Study the drawing (mm; zero at the part's minimum x, y, z) and answer. Give positions to 0.01 mm unless a question says otherwise; leave off trailing zeros. Write each loop counter-clockwise with the first axis right and the second up, starting at its lowest first coordinate (ties: lowest second). Pieces come first, ordered by that corner, then holes. Notation, with made-up numbers: (3, -38) -> (54, -38) arc R16 ccw to (54, -17) -> close; hole circle Ø8 at (44.25, 34.25). An arc over 180 degrees is marked (long way). Put each result on its own line as item: value. Start each with the question number.
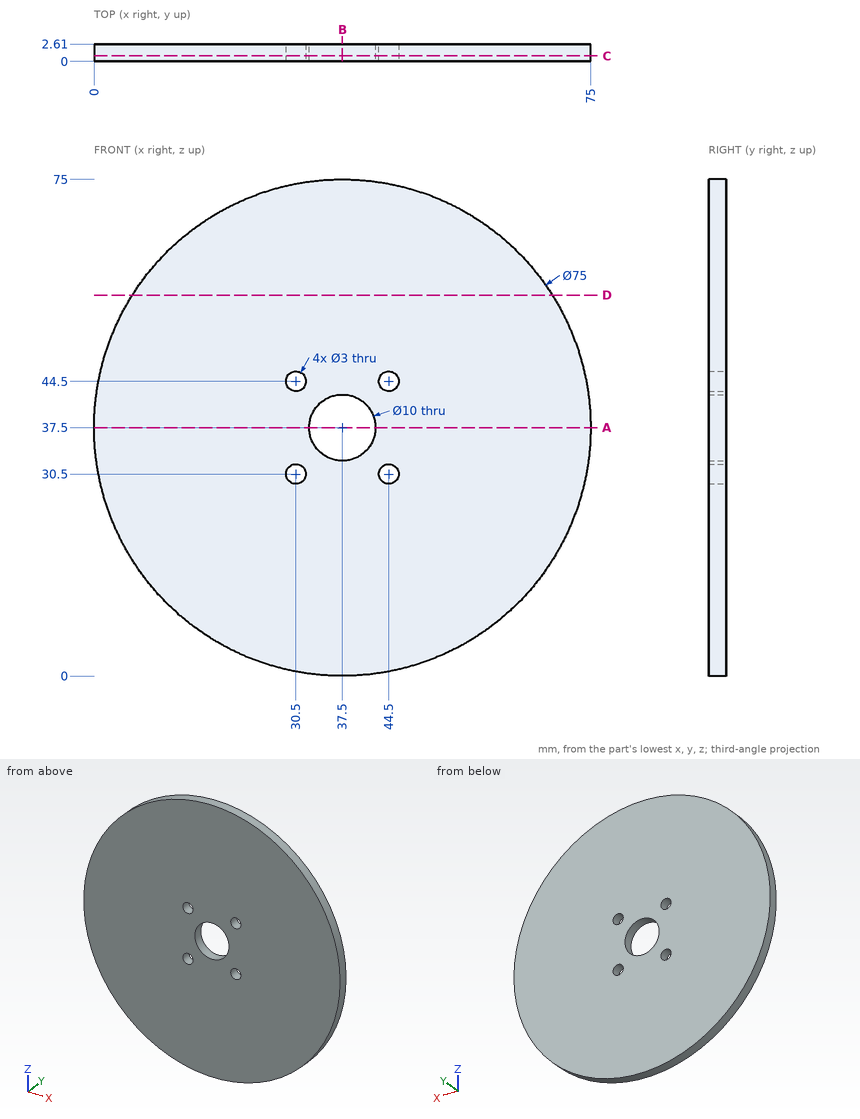
1) A cutting plane is placed at A-A on z = 37.5. Give the vertices of the cut face in (x, y), and give its area (3 significant figures).
2) A cutting plane is placed at C-C on y = 0.8. Give the vertices of the cut face in (x, z), and give its area (3 significant figures).
3) Straight lines are drawn through the part: line 1 (Z direction, x = 30.5, y = 1.15); line 2 (X direction, y = 1.1, z = 37.5). For each, find the intervals that lie inside material, in ascending order. Write a range as [from, to].
4) A cutting plane is placed at D-D on z = 57.5. Give the vertices of the cut face in (x, y), and give its area (3 significant figures).
5) A cutting plane is placed at B-B on x = 37.5. Give the vertices of the cut face in (y, z).
6) Each of these flat-tipped pins is pushed along its axis until it touches: pin 1 Ø1.5 at (y, z) = (2, 56.5) entering from -X; pin 2 Ø1.5 at (x, y) = (16.5, 1.5) entering from -Z; pin 3 Ø1.5 at (y, z) = (1.5, 35.5) entering from -X. Where does it stop, or does it pass through?
Results found:
1. outline: (0, 0) -> (32.5, 0) -> (32.5, 2.61) -> (0, 2.61) -> close; (42.5, 0) -> (75, 0) -> (75, 2.61) -> (42.5, 2.61) -> close
1. area: 170 mm²
2. outline: circle Ø75 at (37.5, 37.5); hole circle Ø3 at (30.5, 30.5); hole circle Ø3 at (30.5, 44.5); hole circle Ø10 at (37.5, 37.5); hole circle Ø3 at (44.5, 30.5); hole circle Ø3 at (44.5, 44.5)
2. area: 4,310 mm²
3. line 1: z = [0.66, 29], [32, 43], [46, 74.34]
3. line 2: x = [0, 32.5], [42.5, 75]
4. outline: (5.78, 0) -> (69.22, 0) -> (69.22, 2.61) -> (5.78, 2.61) -> close
4. area: 166 mm²
5. outline: (0, 0) -> (2.61, 0) -> (2.61, 32.5) -> (0, 32.5) -> close; (0, 42.5) -> (2.61, 42.5) -> (2.61, 75) -> (0, 75) -> close
6. pin 1: stops at x = 4.74
6. pin 2: stops at z = 5.94
6. pin 3: stops at x = 0.02
